Geometry: see drawing. Coordinates: mm, zero at the bounding-box minimum. A direction names the side the tool comes from. Give positions to 0.01 mm unless a question says otherwise; leave off trailing zeros. Write each loop counter-clockwise with the first axis right and the second up, starting at its lowest first coordinate (ties: lowest second). Pieces come first, ordered by that corner, then holes. Notation, with made-up numbers: (11.5, -6.75) - (40.5, -6.75) arc R20 ccw to (40.5, 28.25) - close; hole circle Ø10 at (44, 14.25). An arc over 180 degrees is marked (long way). Use a Markdown table: item, result. Add a question column.
1. Section query C-C, the plane x = 4. Return loops of the section in (y, z), plus the area to 3 significant figures.
2. Section query B-B, the plane y = 1.35. Return loops of the section in (x, z), plus the area to 3 significant figures.
3. Pin query (flat end, axial travel): pin 1 (0.5 mm diameter, centred on y = 3, z = 0.5, fed in from -X); pin 2 (1 mm diameter, centred on y = 3.5, z = 1, fed in from +X). Return the tip coordinate at first contact, or that it passes through.
4. Section query D-D, the plane z = 4.2. Return loops of the section in (x, y), plus the area to 3 significant figures.
5. Mould query, pull axis Z, two halves, no side actions, for the marked faces 1, 2 and 3. Classes: released by +Z, released by -Z, zero draft, split by the parting line, or undercut.
6. Material intervals for probe 1 along Z at (x, y) = (5, 4.15); probe 2 along Z at (x, y) = (2.75, 2.3); probe 3 along X at (y, z) = (0.85, 1.35), sorted ascending.
7. Set-up query: the marked faces 4, 5 and 6. Return all of +Z, -Z, +X, -X, +Y, -Y with unobstructed straight access to the full face (end or side cutting, diameter ignored); none if empty.
8. Section query A-A, the plane x = 6.25. Return loops of the section in (y, z).
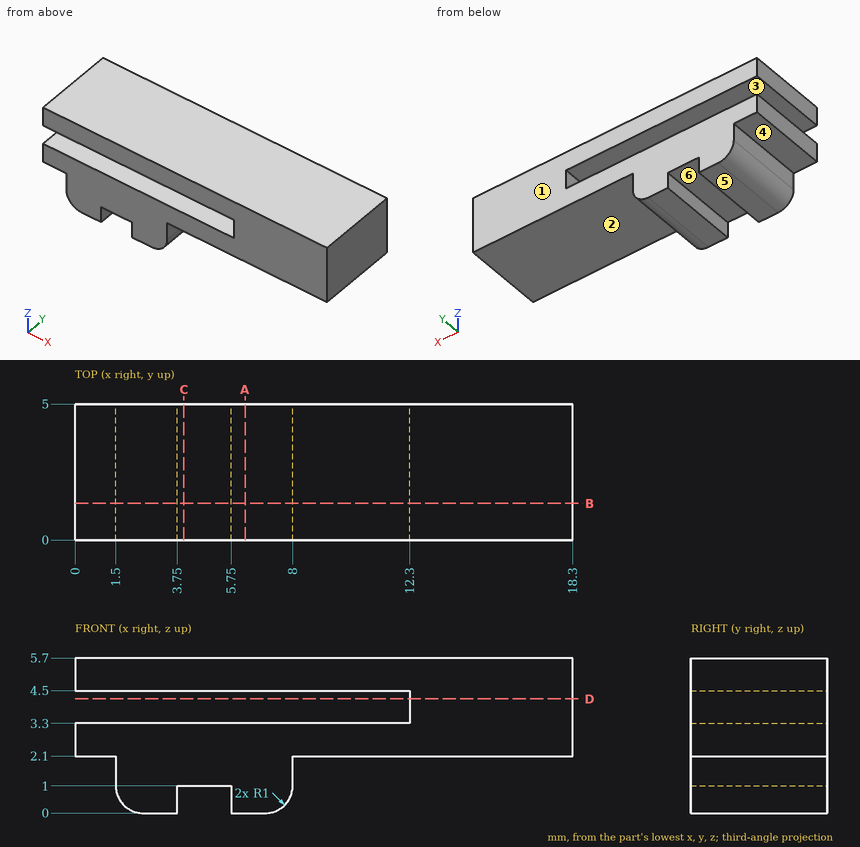
Result sheet:
| question | item | result |
|---|---|---|
| 1 | outline | (0, 1) - (5, 1) - (5, 3.3) - (0, 3.3) - close; (0, 4.5) - (5, 4.5) - (5, 5.7) - (0, 5.7) - close |
| 1 | area | 17.5 mm² |
| 2 | outline | (0, 2.1) - (1.5, 2.1) - (1.5, 1) arc R1 ccw to (2.5, 0) - (3.75, 0) - (3.75, 1) - (5.75, 1) - (5.75, 0) - (7, 0) arc R1 ccw to (8, 1) - (8, 2.1) - (18.3, 2.1) - (18.3, 5.7) - (0, 5.7) - (0, 4.5) - (12.3, 4.5) - (12.3, 3.3) - (0, 3.3) - close |
| 2 | area | 62.3 mm² |
| 3 | pin 1 | stops at x = 1.53 |
| 3 | pin 2 | stops at x = 8 |
| 4 | outline | (12.3, 0) - (18.3, 0) - (18.3, 5) - (12.3, 5) - close |
| 4 | area | 30.0 mm² |
| 5 | face 1 | zero draft |
| 5 | face 2 | released by -Z |
| 5 | face 3 | undercut |
| 6 | probe 1 | z = 1 to 3.3, 4.5 to 5.7 |
| 6 | probe 2 | z = 0 to 3.3, 4.5 to 5.7 |
| 6 | probe 3 | x = 1.5 to 8 |
| 7 | face 4 | -Z, -X, +Y, -Y |
| 7 | face 5 | -Z, +X, -X, +Y, -Y |
| 7 | face 6 | -Z, +Y, -Y |
| 8 | outline | (0, 0) - (5, 0) - (5, 3.3) - (0, 3.3) - close; (0, 4.5) - (5, 4.5) - (5, 5.7) - (0, 5.7) - close |
